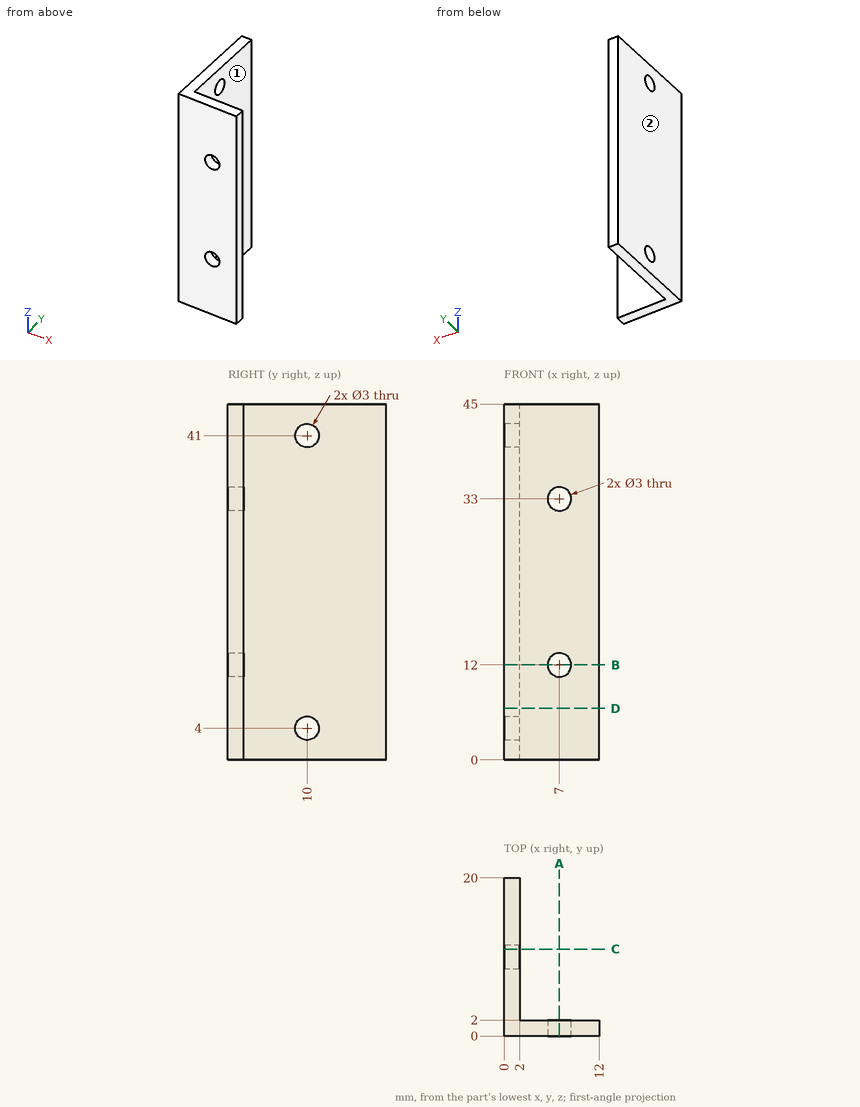
Can you work these out from the drawing? Everything is in mm from the part's minimum corner. A direction names the side the tool comes from. Give positions to 0.01 mm unless a question says otherwise; leave off trailing zeros. Loops run counter-clockwise (first coordinate to the right, second up) from the corner with the lowest first, then second, coordinate; pieces in that order, holes last. Notation, with made-up numbers: (43.25, 1.5) -> (49.25, 1.5) arc R28 ccw to (49.25, 37.5) -> close; hole circle Ø7 at (8, 86.25). An arc over 180 degrees is marked (long way). Put each result on its own line as item: value.
(1) Imagine slicing it at A-A on x = 7. Write out the boundary of the cut face in (y, z).
Computed:
outline: (0, 0) -> (2, 0) -> (2, 10.5) -> (0, 10.5) -> close; (0, 13.5) -> (2, 13.5) -> (2, 31.5) -> (0, 31.5) -> close; (0, 34.5) -> (2, 34.5) -> (2, 45) -> (0, 45) -> close
(2) I'm going to push flat-ended pins straight in: pin 1 Ø1.8 at (y, z) = (10, 4) entering from -X; pin 2 Ø5 at (x, z) = (7, 12) entering from -Y; pin 3 Ø4 at (x, z) = (8, 40) entering from +Y; pin 4 Ø2 at (y, z) = (7.5, 16.5) entering from +X. Where does each tip first touch, or does it pass through?
Computed:
pin 1: through
pin 2: y = 0
pin 3: y = 2
pin 4: x = 2
(3) Please list where these lines run through material, in increasing order: probe 1 along Z at (x, y) = (7, 1.15); probe 2 along Z at (x, y) = (1.75, 9.75); probe 3 along X at (y, z) = (12, 36.5). Write a range as [from, to].
Computed:
probe 1: [0, 10.5], [13.5, 31.5], [34.5, 45]
probe 2: [0, 2.52], [5.48, 39.52], [42.48, 45]
probe 3: [0, 2]
(4) Imagine slicing it at B-B on z = 12. Write out the boundary of the cut face in (x, y), plus the area to 3 significant figures.
Computed:
outline: (0, 0) -> (5.5, 0) -> (5.5, 2) -> (2, 2) -> (2, 20) -> (0, 20) -> close; (8.5, 0) -> (12, 0) -> (12, 2) -> (8.5, 2) -> close
area: 54.0 mm^2
(5) For the marked faces 1 and 2, which set-ups out of +Z, -Z, +X, -X, +Y, -Y let a thin tool reach every point of the face, with its end or its side?
Computed:
face 1: +Z, -Z, +X, +Y
face 2: +Z, -Z, -X, +Y, -Y
(6) Imagine slicing it at C-C on y = 11. Write out the boundary of the cut face in (x, z), plus the area to 3 significant figures.
Computed:
outline: (0, 0) -> (2, 0) -> (2, 2.88) -> (0, 2.88) -> close; (0, 5.12) -> (2, 5.12) -> (2, 39.88) -> (0, 39.88) -> close; (0, 42.12) -> (2, 42.12) -> (2, 45) -> (0, 45) -> close
area: 81.1 mm^2
(7) Imagine slicing it at D-D on z = 6.5. Write out the boundary of the cut face in (x, y).
Computed:
outline: (0, 0) -> (12, 0) -> (12, 2) -> (2, 2) -> (2, 20) -> (0, 20) -> close
